Input: part model. Units: mm. Frame: model coordinates. Give positions to 0.01 mm unless a question says otherwise; leave off trailing zeros. Loops run counter-clockwise (first coordinate to the right, second up) from the corner with the lowest first, then second, coordinate; pieces in that order, holes last. Notation, with made-up numbers: (84.25, -28.5) - (128.25, -28.5) arc R9 cw to (128.25, -17.5) - close; hole circle Ø8 at (11.25, -15.5). An arc over 180 degrees is marked (long way). Answer as a JSON object with one key per item and string values. Group by question number.
(1) Material intervals for L1, parallel to Z at x = 13.25, y = 10.44; L2, parallel to Z at x = 9, y = 15; L3, parallel to Y at x = 13.5, z = 87.3, sorted ascending.
(2) Section query A-A (z = 12.7). Return loops of the section in (x, y).
(3) Section query B-B (y = 10.44). Return loops of the section in (x, z) (1 decimal).
(4) Section query C-C (z = 50). Return loops of the section in (x, y).
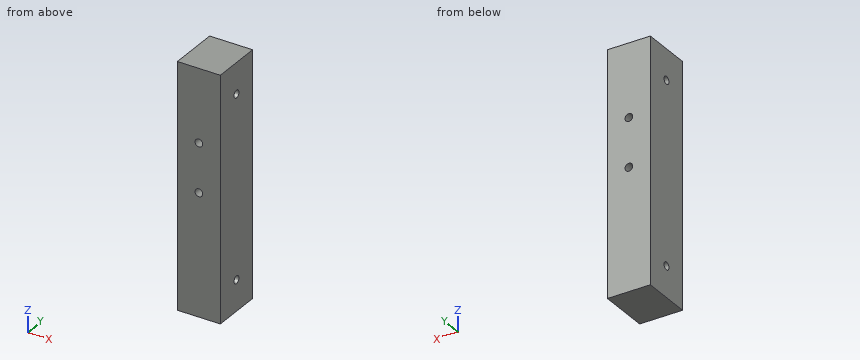
```python
from build123d import *

# Parameters (mm, degrees)
SKETCH1_W           = 17.69
SKETCH1_H           = 20.88
BOSS_EXTRUDE1_DEPTH = 100
SKETCH2_R           = 1.5875
CUT_EXTRUDE1_DEPTH  = 106.78
SKETCH3_R           = 1.5875
CUT_EXTRUDE2_DEPTH  = 100


with BuildPart() as part:
    # Sketch1 → Boss-Extrude1 (new body)
    with BuildSketch(Plane.XY):
        with Locations((8.845, 10.44)):
            Rectangle(SKETCH1_W, SKETCH1_H)
    extrude(amount=BOSS_EXTRUDE1_DEPTH)

    # Sketch2 → Cut-Extrude1 (cut)
    with BuildSketch(Plane(origin=(0, 20.88, 0), x_dir=(1, 0, 0), z_dir=(0, 1, 0))):
        with Locations(Location((8.845, -50, 0), (0, 0, 270))):
            Circle(SKETCH2_R)
        with Locations(Location((8.845, -70, 0), (0, 0, 270))):
            Circle(SKETCH2_R)
    extrude(amount=-CUT_EXTRUDE1_DEPTH, mode=Mode.SUBTRACT)

    # Sketch3 → Cut-Extrude2 (cut)
    with BuildSketch(Plane(origin=(17.69, 0, 0), x_dir=(0, 0, -1), z_dir=(1, 0, 0))):
        with Locations(Location((-87.3, 10.44, 0), (0, 0, 90))):
            Circle(SKETCH3_R)
        with Locations(Location((-12.7, 10.44, 0), (0, 0, 90))):
            Circle(SKETCH3_R)
    extrude(amount=-CUT_EXTRUDE2_DEPTH, mode=Mode.SUBTRACT)


solid = part.part
```
Recorded:
{
 "1": {"L1": "z = 0 to 11.11, 14.29 to 85.71, 88.89 to 100", "L2": "z = 0 to 48.42, 51.58 to 68.42, 71.58 to 100", "L3": "y = 0 to 8.85, 12.03 to 20.88"},
 "2": {"outline": "(0, 0) - (17.69, 0) - (17.69, 8.85) - (0, 8.85) - close; (0, 12.03) - (17.69, 12.03) - (17.69, 20.88) - (0, 20.88) - close"},
 "3": {"outline": "(0, 0) - (17.7, 0) - (17.7, 11.1) - (0, 11.1) - close; (0, 14.3) - (17.7, 14.3) - (17.7, 85.7) - (0, 85.7) - close; (0, 88.9) - (17.7, 88.9) - (17.7, 100) - (0, 100) - close; hole circle Ø3.2 at (8.8, 50); hole circle Ø3.2 at (8.8, 70)"},
 "4": {"outline": "(0, 0) - (7.26, 0) - (7.26, 20.88) - (0, 20.88) - close; (10.43, 0) - (17.69, 0) - (17.69, 20.88) - (10.43, 20.88) - close"}
}
